```python
from build123d import *

# Parameters (mm, degrees)
SKETCH1_W           = 20
SKETCH1_H           = 20
BOSS_EXTRUDE1_DEPTH = 5
SKETCH2_W           = 5
SKETCH2_H           = 20
BOSS_EXTRUDE2_DEPTH = 5
SKETCH3_R           = 10
BOSS_EXTRUDE5_DEPTH = 5
SKETCH6_R           = 10
BOSS_EXTRUDE6_DEPTH = 5
SKETCH5_R           = 4
CUT_EXTRUDE1_DEPTH  = 21


with BuildPart() as part:
    # Sketch1 → Boss-Extrude1 (new body)
    with BuildSketch(Plane.XY):
        with Locations((10, 10)):
            Rectangle(SKETCH1_W, SKETCH1_H)
    extrude(amount=BOSS_EXTRUDE1_DEPTH)

    # Sketch2 → Boss-Extrude2 (add)
    with BuildSketch(Plane.XY.offset(5)):
        with Locations((2.5, 10)):
            Rectangle(SKETCH2_W, SKETCH2_H)
        with Locations((17.5, 10)):
            Rectangle(SKETCH2_W, SKETCH2_H)
    extrude(amount=BOSS_EXTRUDE2_DEPTH)

    # Sketch3 → Boss-Extrude5 (add)
    with BuildSketch(Plane(origin=(20, 0, 0), x_dir=(0, 0, -1), z_dir=(1, 0, 0))):
        with Locations((-10, 10)):
            Circle(SKETCH3_R)
    extrude(amount=-BOSS_EXTRUDE5_DEPTH)

    # Sketch6 → Boss-Extrude6 (add)
    with BuildSketch(Plane.ZY):
        with Locations((10, 10)):
            Circle(SKETCH6_R)
    extrude(amount=-BOSS_EXTRUDE6_DEPTH)

    # Sketch5 → Cut-Extrude1 (cut, through all)
    with BuildSketch(Plane(origin=(20, 0, 0), x_dir=(0, 0, -1), z_dir=(1, 0, 0))):
        with Locations((-10, 10)):
            Circle(SKETCH5_R)
    extrude(amount=-CUT_EXTRUDE1_DEPTH, mode=Mode.SUBTRACT)


solid = part.part
```
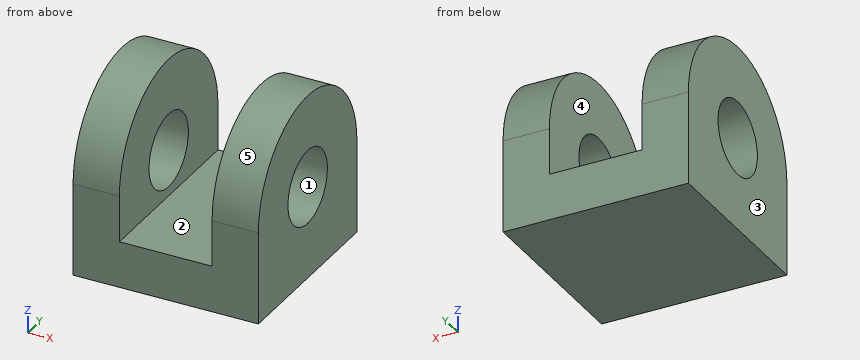
Could you check a few things on this model? Use its own coordinates, in mm. Face numbers are marked on the shaded views. A direction names the side the tool comes from. Coordinates: 2 decimals unless noted, no trailing zeros. Loops run counter-clockwise (first coordinate to the right, second up) from the corner with the lowest first, then second, coordinate; pieces in that order, holes last. Notation, with made-up numbers: M 23.25,35.5 L 81.25,35.5 A23 cw 81.25,60.5 Z; hole C 6,-22 d3. An arc over 180 degrees is marked long. Put each result on its own line as item: value. Start each with the question number.
(1) I need wall thicknesses on line 1 (X direction, y = 3.5, z = 9); line 2 (Y direction, x = 17.7, z = 10); line 3 (Z direction, x = 6, y = 8.75). Which ranges of each line are inside material? Lowest first, please. Write a range as from..to.
(2) For the marked faces 1 and 2, which set-ups out of +Z, -Z, +X, -X, +Y, -Y let a thin tool reach every point of the face, with its end or its side?
(3) Suppose I cut it at D-D on z = 10.75. Please give me the cut outline in (x, y), then the cut area to 3 significant figures.
(4) Will these pins go through, and if not, where does the flat tip stop? P1, Ø3, axis at x = 3, z = 15, coming from the -Y side; P2, Ø7, axis at y = 10, z = 10, coming from the -X side; P3, Ø8, axis at x = 2.5, z = 16, coming from the -Y side; P4, Ø5, axis at x = 8.5, y = 13, coming from the +Z side.
(5) Suppose I cut it at C-C on z = 17. Please give me the cut outline in (x, y).
(6) Suppose I cut it at B-B on x = 4.5. Please give me the cut outline in (y, z), then the cut area to 3 significant figures.
(7) Suppose I cut it at A-A on y = 10. Please give me the cut outline in (x, z).
(8) Thinking about a two-plate mould opening in X: for the marked faces 3, 4 and 5, which applies, pulls with the +X half, pulls with the -X half, needs draft (parallel to the pull), parting line crosses it, or undercut?
Solutions:
1. line 1: x = 0..5, 15..20
1. line 2: y = 0..6, 14..20
1. line 3: z = 0..5
2. face 1: +X, -X
2. face 2: +Z, +Y, -Y
3. outline: M 0,0.03 L 5,0.03 L 5,6.07 L 0,6.07 Z; M 0,13.93 L 5,13.93 L 5,19.97 L 0,19.97 Z; M 15,0.03 L 20,0.03 L 20,6.07 L 15,6.07 Z; M 15,13.93 L 20,13.93 L 20,19.97 L 15,19.97 Z
3. area: 121 mm2
4. P1: stops at y = 0.63
4. P2: passes through
4. P3: stops at y = 0.2
4. P4: stops at z = 5
5. outline: M 0,2.86 L 5,2.86 L 5,17.14 L 0,17.14 Z; M 15,2.86 L 20,2.86 L 20,17.14 L 15,17.14 Z
6. outline: M 0,0 L 20,0 L 20,10 A10 ccw 0,10 Z; hole C 10,10 d8
6. area: 307 mm2
7. outline: M 0,0 L 20,0 L 20,6 L 15,6 L 15,5 L 5,5 L 5,6 L 0,6 Z; M 0,14 L 5,14 L 5,20 L 0,20 Z; M 15,14 L 20,14 L 20,20 L 15,20 Z
8. face 3: pulls with the -X half
8. face 4: undercut
8. face 5: needs draft
